Geometry check sheet. Reference: the model listing, model coordinates, mm. A direction names the side the tool comes from. Round coordinates to 2 decimals unless told otherwise and drop trailing zeros. Order: outer loops, then holes, each group sorted by start corner. A loop starts at its lowest first (then second) coordinate and runs counter-clockwise, first axis right, second up.
(1) Thickness scan on L1, parallel to Z at x = 82, y = 6; L2, parallel to X at y = 18, z = 27.5; L3, parallel to X at y = 13.75, z = 17.5. Record the ranges inside material, lowest first.
(2) Draft check along X on faces 4 (the face through (178.841, 16.262, -16.987)), 5 (the face through (101.52, 0, 77.35)), 6 (the face through (97.15, 9.86, 81.19)), 7 (the face through (93.581, 12.325, 99.887)). Enter one of: pulls with the +X half, pulls with the -X half, needs draft (parallel to the pull), parting line crosses it, or undercut.
(3) Set-up check for faces 1 (the face through (90, 22, 85)), 2 (the face through (83, 0, 99)), 3 (the face through (1.051, 17.188, 11.536)): record each of +Z, -Z, +X, -X, +Y, -Y from which the full face is reachable in a straight line by a thin tool's end or side.
(4) Gauge pin test, flat ends, axial feed: P1, Ø10, axis at x = 95.5, y = 10.5, coming from the +Z side; P2, Ø12, axis at x = 55.5, z = 86.5, coming from the -Y side; P3, Ø5, axis at x = 156, y = 6, coming from the +Z side. Record the tip position at first contact, or that the pin passes through.
(5) Cross-section at A-A on x = 82.5. Enter the section's corners in (y, z), and give its area (3 significant figures).
Autodesk Inventor part; units mm, degrees
ref_plane "YZ Plane" through (0, 0, 0) normal (1, 0, 0) x (0, 1, 0)
ref_plane "XZ Plane" through (0, 0, 0) normal (0, 1, 0) x (-1, 0, 0)
ref_plane "XY Plane" through (0, 0, 0) normal (0, 0, 1) x (1, 0, 0)
sketch "Sketch1" plane through (0, 0, 0) normal (0, 0, 1) x (1, 0, 0)
  line L0 (-15, 0) -> (-15, 20)
  line L1 (-13, 22) -> (-2, 22)
  line L2 (0, 20) -> (0, 0)
  line L3 (0, 0) -> (3, 0)
  line L4 (3, 0) -> (3, 25)
  line L5 (3, 25) -> (-18, 25)
  line L6 (-18, 25) -> (-18, 0)
  line L7 (-18, 0) -> (-15, 0)
  line L8 (82.5, 0) -> (82.5, 23.5159) construction
  arc A0 (0, 20) -> (-2, 22) centre (-2, 20) ccw
  arc A1 (-13, 22) -> (-15, 20) centre (-13, 20) ccw
  point P0 (-15, 22)
  point P1 (0, 22)
  point P2 (-7.5, 0)
  dimension "d0" = 22
  dimension "d2" = 15
  dimension "d3" = 3
  dimension "d4" = 25
  dimension "d5" = 21
  dimension "d6" = 7.5
  dimension "d7" = 0
  dimension "d8" = 90
  dimension "d9" = 2
  dimension "d15" = 0
revolve "Revolution1" add sketch "Sketch1" angle 190 about axis through (82.5, 0, 0) along (0, 1, 0)
sketch "Sketch2" plane through (-18, 25, 0) normal (0, 1, 0) x (1, 0, 0)
  arc A0 (21, 0) -> (178.7922, 13.805) centre (100.5, 0) ccw
  arc A1 (3, 0) -> (196.5188, 16.9307) centre (100.5, 0) ccw
  line L0 (100.5, 0) -> (3, 0)
  line L1 (5, 0) -> (16, 0)
  line L2 (100.5, 0) -> (22.2078, -13.805)
  line L3 (22.2078, -13.805) -> (3, 0)
  point P0 (18, 0)
  point P1 (21, 0)
  dimension "d12" = 10
extrude "Extrusion1" cut sketch "Sketch2" against normal up to surface (25 mm away) contours A0 L3 L0
properties part number "InertiaKitOuter"
Found:
1. L1: z = 79.5 to 82.5, 97.5 to 100.5
1. L2: x = -14.16 to -11.04, 4.72 to 7.91, 157.09 to 160.28, 176.04 to 179.16
1. L3: x = -16.46 to -13.42, 1.88 to 4.95, 160.05 to 163.12, 178.42 to 181.46
2. face 4: pulls with the -X half
2. face 5: needs draft
2. face 6: undercut
2. face 7: parting line crosses it
3. face 1: -Y
3. face 2: +Z, -Z, +X, -X, -Y
3. face 3: -Z, +Y, -Y
4. P1: stops at z = 100.18
4. P2: stops at y = 21.66
4. P3: stops at z = 71.13
5. outline: (0, 79.5) - (25, 79.5) - (25, 100.5) - (0, 100.5) - (0, 97.5) - (20, 97.5) arc R2 cw to (22, 95.5) - (22, 84.5) arc R2 cw to (20, 82.5) - (0, 82.5) - close
5. area: 197 mm2
